Here's how the part is built. I have some questions about the finished solid (model axes, mm). Coordinates: 2 decimals unless noted, no trailing zeros. Loops run counter-clockwise (first coordinate to the right, second up) from the corner with the lowest first, then second, coordinate; pieces in that order, holes last. Notation, with made-up numbers: (73, -11) -> (126, -11) arc R26 cw to (126, 25) -> close; hole circle Ø11 at (18.5, 14.25). An arc over 180 degrees is marked (long way). Answer as a JSON object with one key per item and string values. Group by question number.
1) I'm going to push a flat-ended pin straight in: pin 1 (4 mm diameter, centred on x = 10, y = 10, fed in from -Z). Where does the tip first touch, or does it pass through?
2) I want a section at B-B (x = 74). Write out the boundary of the cut face in (y, z).
3) I want a section at A-A (x = 170). Write out the boundary of the cut face in (y, z).
4) I need wall thicknesses on probe 1 along Y at (x, z) = (10, 1.3); probe 2 along Y at (x, z) = (74, 0.95); probe 3 along X at (y, z) = (8.5, 0.7). Which ranges of each line are inside material? Lowest first, please. Write a range as [from, to].
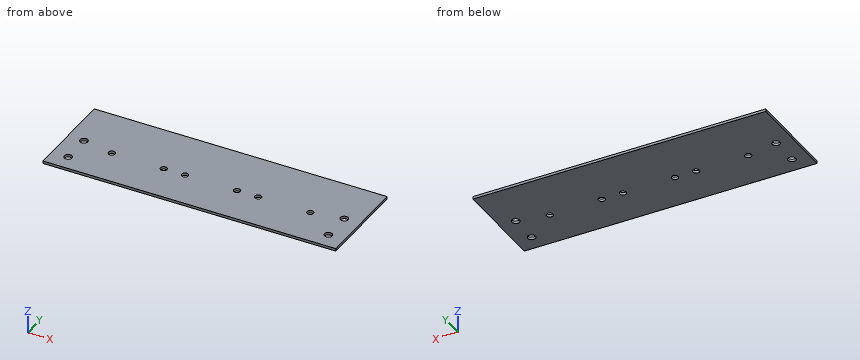
```python
from build123d import *

# Parameters (mm, degrees)
SKETCH1_W           = 180
SKETCH1_H           = 58
SKETCH1_R           = 2.35
SKETCH1_R_2         = 2
BOSS_EXTRUDE1_DEPTH = 1.6


with BuildPart() as part:
    # Sketch1 → Boss-Extrude1 (new body)
    with BuildSketch(Plane.XY):
        with Locations((90, 29)):
            Rectangle(SKETCH1_W, SKETCH1_H)
        with Locations((10, 28)):
            Circle(SKETCH1_R, mode=Mode.SUBTRACT)
        with Locations((10, 10)):
            Circle(SKETCH1_R, mode=Mode.SUBTRACT)
        with Locations((29, 24.5)):
            Circle(SKETCH1_R_2, mode=Mode.SUBTRACT)
        with Locations((61, 24.5)):
            Circle(SKETCH1_R_2, mode=Mode.SUBTRACT)
        with Locations((74, 24.5)):
            Circle(SKETCH1_R_2, mode=Mode.SUBTRACT)
        with Locations((106, 24.5)):
            Circle(SKETCH1_R_2, mode=Mode.SUBTRACT)
        with Locations((119, 24.5)):
            Circle(SKETCH1_R_2, mode=Mode.SUBTRACT)
        with Locations((151, 24.5)):
            Circle(SKETCH1_R_2, mode=Mode.SUBTRACT)
        with Locations((170, 28)):
            Circle(SKETCH1_R, mode=Mode.SUBTRACT)
        with Locations((170, 10)):
            Circle(SKETCH1_R, mode=Mode.SUBTRACT)
    extrude(amount=BOSS_EXTRUDE1_DEPTH)


solid = part.part
```
Determined:
{
 "1": {"pin 1": "through"},
 "2": {"outline": "(0, 0) -> (22.5, 0) -> (22.5, 1.6) -> (0, 1.6) -> close; (26.5, 0) -> (58, 0) -> (58, 1.6) -> (26.5, 1.6) -> close"},
 "3": {"outline": "(0, 0) -> (7.65, 0) -> (7.65, 1.6) -> (0, 1.6) -> close; (12.35, 0) -> (25.65, 0) -> (25.65, 1.6) -> (12.35, 1.6) -> close; (30.35, 0) -> (58, 0) -> (58, 1.6) -> (30.35, 1.6) -> close"},
 "4": {"probe 1": "[0, 7.65], [12.35, 25.65], [30.35, 58]", "probe 2": "[0, 22.5], [26.5, 58]", "probe 3": "[0, 8.19], [11.81, 168.19], [171.81, 180]"}
}
